from build123d import *

# Parameters (mm, degrees)
F0_W     = 63.5
F0_H     = 63.5
F1_DEPTH = 38.1
F2_R     = 5.08


with BuildPart() as f1:
    # F0 (on Front) → F1 (new body)
    with BuildSketch(Plane.XZ):
        with Locations((31.75, 31.75)):
            Rectangle(F0_W, F0_H)
        with BuildLine():
            ThreePointArc((19.05, 12.7), (13.648367, 15.711607), (13.370387, 21.889806))
            Line((13.370387, 21.889806), (26.070387, 47.289806))
            ThreePointArc((26.070387, 47.289806), (31.75, 50.8), (37.429613, 47.289806))
            Line((37.429613, 47.289806), (50.129613, 21.889806))
            ThreePointArc((50.129613, 21.889806), (49.851633, 15.711607), (44.45, 12.7))
            Line((44.45, 12.7), (19.05, 12.7))
        make_face(mode=Mode.SUBTRACT)
    extrude(amount=F1_DEPTH)

    # F2
    f2_edges = [f1.edges().sort_by_distance(p)[0] for p in [
        (31.75, -38.1, 63.5),
        (63.5, -19.05, 63.5),
        (31.75, 0, 63.5),
        (0, -19.05, 63.5),
        (0, 0, 31.75),
        (0, -38.1, 31.75),
        (0, -19.05, 0),
        (31.75, 0, 0),
        (31.75, -38.1, 0),
        (63.5, -19.05, 0),
        (63.5, 0, 31.75),
        (63.5, -38.1, 31.75),
    ]]
    fillet(f2_edges, radius=F2_R)


solid = f1.part
Geometry check sheet. Reference: the model listing, model coordinates, mm. A direction names the side the tool comes from. Give positions to 0.01 mm unless a question says otherwise; leave off trailing zeros. Write each loop counter-clockwise with the first axis right and the second up, starting at its lowest first coordinate (ties: lowest second). Pieces come first, ordered by that corner, then holes. Notation, with made-up numbers: M 85,71.25 L 114,71.25 A34 ccw 114,110.25 Z; hole C 42,59 d2. An arc over 180 degrees is marked long. One line per question, with ' | ' between items.
1. Cross-section at D-D (y = -35). Enter the section's corners in (x, z), plus the area to 3 significant figures.
Ans:
outline: M 0.4,5.08 A4.68 ccw 5.08,0.4 L 58.42,0.4 A4.68 ccw 63.1,5.08 L 63.1,58.42 A4.68 ccw 58.42,63.1 L 5.08,63.1 A4.68 ccw 0.4,58.42 Z; hole M 13.37,21.89 A6.35 ccw 19.05,12.7 L 44.45,12.7 A6.35 ccw 50.13,21.89 L 37.43,47.29 A6.35 ccw 26.07,47.29 Z | area: 2,940 mm2
2. Cross-section at B-B (y = -20). Enter the section's corners in (x, z), plus the area to 3 significant figures.
Ans:
outline: M 0,5.08 A5.08 ccw 5.08,0 L 58.42,0 A5.08 ccw 63.5,5.08 L 63.5,58.42 A5.08 ccw 58.42,63.5 L 5.08,63.5 A5.08 ccw 0,58.42 Z; hole M 13.37,21.89 A6.35 ccw 19.05,12.7 L 44.45,12.7 A6.35 ccw 50.13,21.89 L 37.43,47.29 A6.35 ccw 26.07,47.29 Z | area: 3,040 mm2
3. Set-up check for faces 1 (the face through (1.449, -19.246, 1.528)), 2 (the face through (32, -19, 12.7)): record each of +Z, -Z, +X, -X, +Y, -Y from which the full face is reachable in a straight line by a thin tool's end or side.
Ans:
face 1: -Z, -X, +Y, -Y | face 2: +Y, -Y
4. Cross-section at C-C (x = 33). Enter the section's corners in (y, z).
Ans:
outline: M -38.1,5.08 A5.08 ccw -33.02,0 L -5.08,0 A5.08 ccw 0,5.08 L 0,12.7 L -38.1,12.7 Z; M -38.1,50.68 L 0,50.68 L 0,58.42 A5.08 ccw -5.08,63.5 L -33.02,63.5 A5.08 ccw -38.1,58.42 Z
5. Mould release check, pull along X, two halves, no side actions. Record for faces 3 (the face through (63.5, -19, 31)), 4 (the face through (49.9, -18.78, 15.79)), 5 (the face through (43, 0, 38)): released by +X, released by -X, zero draft, split by the parting line, or undercut.
Ans:
face 3: released by +X | face 4: undercut | face 5: zero draft
6. Cross-section at A-A (z = 15). Enter the section's corners in (x, y), plus the area to 3 significant figures.
Ans:
outline: M 0,-33.02 A5.08 ccw 5.08,-38.1 L 14.16,-38.1 L 14.16,0 L 5.08,0 A5.08 ccw 0,-5.08 Z; M 49.34,-38.1 L 58.42,-38.1 A5.08 ccw 63.5,-33.02 L 63.5,-5.08 A5.08 ccw 58.42,0 L 49.34,0 Z | area: 1,060 mm2
7. Scan lines: line 1 along X through (y, z) = (-5.5, 19.5); line 2 along Y through (x, z) = (12, 58.5); line 3 along Z through (x, y) = (26, -18). Record each from-to range of solid material in increasing order. Write a range as from..to.
Ans:
line 1: 0..12.72, 50.78..63.5 | line 2: -38.1..0 | line 3: 0..12.7, 47.15..63.5
